Part model, mm, in its own coordinate system. A direction names the side the tool comes from. Give positions to 0.01 mm unless a question says otherwise; leave off trailing zeros. Order: outer loops, then holes, each group sorted by start corner. A loop starts at its lowest first (then second) coordinate and runs counter-clockwise, first axis right, second up. Notation, with made-up numbers: (-22.75, 79) -> (-2.75, 79) arc R12 ccw to (-2.75, 94) -> close; hole circle Ø2 at (-35.5, 52). An arc over 180 degrees is marked (long way). Write item = value, one per line. Start each with the question number.
(1) Which spindle directions (+Z, -Z, +X, -X, +Y, -Y) get a long thin tool onto all of the face, cutting with end or side? Do faces 1 (the flat face through (26, 5, 7.5)), 2 (the flat face through (-11, -13, 15)), 3 (the flat face through (11, -13, 15)), 4 (the flat face through (15, 12, 27)), 5 (the flat face through (0, -17.5, 15)). Say none if no direction does.
(2) Two-plate mould, pull along X, no slides. Class faces 6 (the flat face through (0, 4, 30)), 7 (the flat face through (-35, 11, 15)), 8 (the flat face through (0, 7.5, 27)), 9 (the flat face through (35, 5, 26)): pulls with the +X half, pulls with the -X half, needs draft (parallel to the pull), parting line crosses it, or undercut.
(3) Saw through at C-C, the plane z = 4.5. List the corners of the cut face in (x, y).
(4) Saw through at D-D, the plane z = 15. List the corners of the cut face in (x, y), then the cut area to 3 significant figures.
(5) Saw through at A-A, the plane x = 23.5. List the corners of the cut face in (y, z).
(6) Saw through at B-B, the plane y = -0.5. List the corners of the cut face in (x, z), then the cut area to 3 significant figures.
(7) Probe line 1 along Z through (x, y) = (26, 4); line 2 along Y through (x, z) = (-45, 20); line 3 along X through (y, z) = (-5.5, 5). List the from-to ranges inside material, lowest first. Write a range as from..to.
(8) Flat gauge pins, fed straight in: pin 1 (5 mm diameter, centred on x = 7, y = 14.5, fed in from +Z); pin 2 (3.5 mm diameter, centred on x = -1.5, z = 25.5, fed in from +Y); pin 3 (5 mm diameter, centred on y = -11.5, z = 22.5, fed in from +X). Where does each tip first touch, or does it go through?
from build123d import *

# Parameters (mm, degrees)
SKETCH_1_W               = 22
SKETCH_1_H               = 10
SKETCH_1_W_2             = 16
SKETCH_1_H_2             = 8
EXTRUDE_1_DEPTH          = 30
CUT_EXTRUDE_1_DEPTH      = 30
CUT_EXTRUDE_1_DEPTH_BACK = 30
SKETCH_2_W               = 17
SKETCH_2_H               = 15
SKETCH_3_W               = 30
SKETCH_3_H               = 10
CUT_EXTRUDE_2_DEPTH      = 7


with BuildPart() as part:
    # Эскиз1 → Бобышка-Вытянуть1 (new body)
    with BuildSketch(Plane.XY):
        Polygon((-35, -7.5), (-11, -7.5), (11, -7.5), (35, -7.5), (35, 17.5), (-35, 17.5), (-35, 4), (-35, -4), align=None)
        with Locations((0, -12.5)):
            Rectangle(SKETCH_1_W, SKETCH_1_H)
        with Locations((-43, 0)):
            Rectangle(SKETCH_1_W_2, SKETCH_1_H_2)
    extrude(amount=EXTRUDE_1_DEPTH)

    # Эскиз2 → Вырез-Вытянуть1 (cut, two sides: drawn at the far end of the back side and taken through both)
    with BuildSketch(Plane.XZ.offset(4).offset(-CUT_EXTRUDE_1_DEPTH_BACK)):
        with Locations((26.5, 15)):
            Rectangle(SKETCH_2_W, SKETCH_2_H)
        Polygon((-35, 30), (-51, 30), (-51, 23), align=None)
    extrude(amount=CUT_EXTRUDE_1_DEPTH + CUT_EXTRUDE_1_DEPTH_BACK, mode=Mode.SUBTRACT)

    # Эскиз3 → Вырез-Вытянуть2 (cut)
    with BuildSketch(Plane.XY.offset(30)):
        with Locations((0, 12.5)):
            Rectangle(SKETCH_3_W, SKETCH_3_H)
    extrude(amount=-CUT_EXTRUDE_2_DEPTH, mode=Mode.SUBTRACT)


solid = part.part
Results list:
q1.face_1 = +X, +Y, -Y
q1.face_2 = +Z, -Z, -X, -Y
q1.face_3 = +Z, -Z, +X, -Y
q1.face_4 = +Z, +Y
q1.face_5 = +Z, -Z, +X, -X, -Y
q2.face_6 = needs draft
q2.face_7 = pulls with the -X half
q2.face_8 = undercut
q2.face_9 = pulls with the +X half
q3.outline = (-51, -4) -> (-35, -4) -> (-35, -7.5) -> (-11, -7.5) -> (-11, -17.5) -> (11, -17.5) -> (11, -7.5) -> (35, -7.5) -> (35, 17.5) -> (-35, 17.5) -> (-35, 4) -> (-51, 4) -> close
q4.outline = (-51, -4) -> (-35, -4) -> (-35, -7.5) -> (-11, -7.5) -> (-11, -17.5) -> (11, -17.5) -> (11, -7.5) -> (18, -7.5) -> (18, 17.5) -> (-35, 17.5) -> (-35, 4) -> (-51, 4) -> close
q4.area = 1,670 mm^2
q5.outline = (-7.5, 0) -> (17.5, 0) -> (17.5, 7.5) -> (-7.5, 7.5) -> close; (-7.5, 22.5) -> (17.5, 22.5) -> (17.5, 30) -> (-7.5, 30) -> close
q6.outline = (-51, 0) -> (35, 0) -> (35, 7.5) -> (18, 7.5) -> (18, 22.5) -> (35, 22.5) -> (35, 30) -> (-35, 30) -> (-51, 23) -> close
q6.area = 2,270 mm^2
q7.line_1 = 0..7.5, 22.5..30
q7.line_2 = -4..4
q7.line_3 = -35..35
q8.pin_1 = 23
q8.pin_2 = 7.5
q8.pin_3 = 11
